Source: CAD feature listing. Evaluate the final solid. Frame: model axes, mm. Face numbers are marked on the shaded views. A direction names the side the tool comes from. Coordinates: 2 decimals unless noted, no trailing zeros. Loops run counter-clockwise (first coordinate to the right, second up) from the corner with the lowest first, then second, coordinate; pieces in that order, holes last. Notation, with made-up numbers: (71, 41.25) -> (85, 41.25) arc R10 cw to (85, 50.25) -> close; hole circle Ø8 at (22, 17). An arc over 180 degrees is marked (long way). One line per question, with ' | ' between items. Start each with the question number.
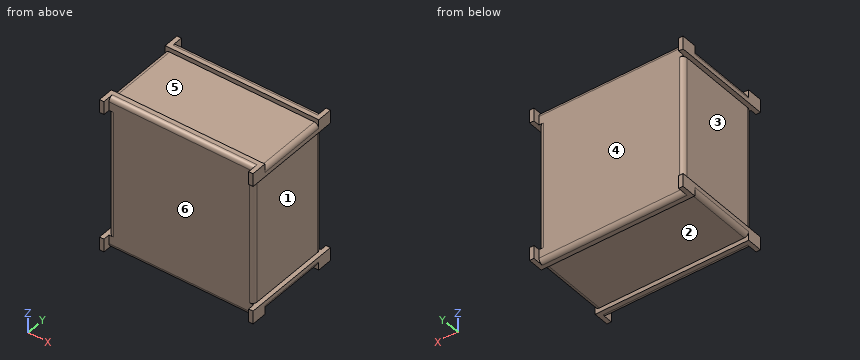
```python
from build123d import *

# Parameters (mm, degrees)
BOSS_EXTRUDE1_DEPTH = 23
CUT_EXTRUDE1_DEPTH  = 1.5
CUT_EXTRUDE2_DEPTH  = 1.5
FILLET2_R           = 1
FILLET3_R           = 1
FILLET4_R           = 1
FILLET5_R           = 1
CUT_EXTRUDE3_DEPTH  = 1
FILLET6_R           = 1
FILLET7_R           = 1
SKETCH6_W           = 35
SKETCH6_H           = 16.000000000000004
CUT_EXTRUDE4_DEPTH  = 1
FILLET8_R           = 1
FILLET9_R           = 1
CUT_EXTRUDE5_DEPTH  = 1
CUT_EXTRUDE6_DEPTH  = 1
FILLET10_R          = 1
FILLET11_R          = 1
FILLET12_R          = 1
FILLET13_R          = 1


with BuildPart() as part:
    # Sketch1 → Boss-Extrude1 (new body)
    with BuildSketch(Plane(origin=(0, 0, 0), x_dir=(1, 0, 0), z_dir=(0, 1, 0))):
        Polygon((-13.200362647325472, 10.07479601087942), (21.799637352674534, 10.07479601087942), (21.799637352674537, -24.925203989120583), (-13.200362647325466, -24.925203989120583), align=None)
    extrude(amount=BOSS_EXTRUDE1_DEPTH)

    # Sketch2 → Cut-Extrude1 (cut)
    with BuildSketch(Plane(origin=(0, 23, 0), x_dir=(1, 0, 0), z_dir=(0, 1, 0))):
        Polygon((20.79963735267453, -24.925203989120583), (-12.200362647325468, -24.925203989120586), (-12.20036264732547, 10.074796010879416), (20.79963735267453, 10.07479601087942), align=None)
    extrude(amount=-CUT_EXTRUDE1_DEPTH, mode=Mode.SUBTRACT)

    # Sketch3 → Cut-Extrude2 (cut)
    with BuildSketch(Plane.XZ):
        Polygon((20.799637352674537, -10.07479601087942), (-12.200362647325464, -10.074796010879423), (-12.200362647325463, 24.92520398912058), (20.799637352674537, 24.925203989120583), align=None)
    extrude(amount=-CUT_EXTRUDE2_DEPTH, mode=Mode.SUBTRACT)

    # Fillet2
    fillet2_edges = [part.edges().sort_by_distance(p)[0] for p in [
        (4.29963735267453, 21.5, -10.074796010879417),
    ]]
    fillet(fillet2_edges, radius=FILLET2_R)

    # Fillet3
    fillet3_edges = [part.edges().sort_by_distance(p)[0] for p in [
        (4.29963735267453, 21.5, 24.925203989120583),
    ]]
    fillet(fillet3_edges, radius=FILLET3_R)

    # Fillet4
    fillet4_edges = [part.edges().sort_by_distance(p)[0] for p in [
        (4.299637352674537, 1.5, 24.925203989120583),
    ]]
    fillet(fillet4_edges, radius=FILLET4_R)

    # Fillet5
    fillet5_edges = [part.edges().sort_by_distance(p)[0] for p in [
        (4.299637352674537, 1.5, -10.074796010879421),
    ]]
    fillet(fillet5_edges, radius=FILLET5_R)

    # Sketch5 → Cut-Extrude3 (cut)
    with BuildSketch(Plane(origin=(0, 0, -10.07479601087942), x_dir=(-1, 0, 0), z_dir=(0, 0, -1))):
        Polygon((13.200362647325472, 3.5089999999999977), (-21.799637352674534, 3.5089999999999937), (-21.799637352674534, 19.508999999999997), (13.200362647325472, 19.509), align=None)
    extrude(amount=-CUT_EXTRUDE3_DEPTH, mode=Mode.SUBTRACT)

    # Fillet6
    fillet6_edges = [part.edges().sort_by_distance(p)[0] for p in [
        (-13.200362647325472, 11.508999999999999, -9.07479601087942),
    ]]
    fillet(fillet6_edges, radius=FILLET6_R)

    # Fillet7
    fillet7_edges = [part.edges().sort_by_distance(p)[0] for p in [
        (21.799637352674534, 11.508999999999995, -9.07479601087942),
    ]]
    fillet(fillet7_edges, radius=FILLET7_R)

    # Sketch6 → Cut-Extrude4 (cut)
    with BuildSketch(Plane.XY.offset(24.925203989120583)):
        with Locations((4.299637352674536, 11.508999999999999)):
            Rectangle(SKETCH6_W, SKETCH6_H)
    extrude(amount=-CUT_EXTRUDE4_DEPTH, mode=Mode.SUBTRACT)

    # Fillet8
    fillet8_edges = [part.edges().sort_by_distance(p)[0] for p in [
        (-13.200362647325463, 11.509, 23.925203989120583),
    ]]
    fillet(fillet8_edges, radius=FILLET8_R)

    # Fillet9
    fillet9_edges = [part.edges().sort_by_distance(p)[0] for p in [
        (21.799637352674537, 11.508999999999999, 23.925203989120583),
    ]]
    fillet(fillet9_edges, radius=FILLET9_R)

    # Sketch7 → Cut-Extrude5 (cut)
    with BuildSketch(Plane(origin=(21.799637352674537, 0, -4.32e-15), x_dir=(-2e-16, 0, -1), z_dir=(1, 0, -2e-16))):
        Polygon((7.074796010879417, -1.2e-16), (-21.925203989120586, -3.95e-15), (-21.925203989120586, 22.999999999999996), (7.074796010879417, 22.999999999999996), align=None)
    extrude(amount=-CUT_EXTRUDE5_DEPTH, mode=Mode.SUBTRACT)

    # Sketch8 → Cut-Extrude6 (cut)
    with BuildSketch(Plane(origin=(-13.200362647325473, 0, -13.200362647325468), x_dir=(-1.5e-16, 0, -1), z_dir=(1, 0, -1.5e-16))):
        Polygon((-6.125566636446044, 8e-17), (-35.125566636446045, -3.47e-15), (-35.125566636446045, 22.999999999999996), (-6.1255666364460435, 23), align=None)
    extrude(amount=CUT_EXTRUDE6_DEPTH, mode=Mode.SUBTRACT)

    # Fillet10
    fillet10_edges = [part.edges().sort_by_distance(p)[0] for p in [
        (-12.20036264732547, 21.5, 7.425203989120572),
    ]]
    fillet(fillet10_edges, radius=FILLET10_R)

    # Fillet11
    fillet11_edges = [part.edges().sort_by_distance(p)[0] for p in [
        (-12.200362647325463, 1.5, 7.425203989120577),
    ]]
    fillet(fillet11_edges, radius=FILLET11_R)

    # Fillet12
    # the kernel refuses this fillet: 1 mm, written as the material it takes off along each edge
    with BuildSketch(Plane(origin=(20.79963735267453, 21.5, -7.074796010879421), x_dir=(-1, 0, 0), z_dir=(0, 0, 1))) as fillet12_piece_1:
        with BuildLine():
            CenterArc((FILLET12_R, FILLET12_R), FILLET12_R, 180, 90)
            Line((0, FILLET12_R), (0, 0))
            Line((0, 0), (FILLET12_R, 0))
        make_face()
    extrude(amount=29.000000000000004, mode=Mode.SUBTRACT)

    # Fillet13
    # the kernel refuses this fillet: 1 mm, written as the material it takes off along each edge
    with BuildSketch(Plane(origin=(20.799637352674537, 1.5, 21.925203989120583), x_dir=(-1, 0, 0), z_dir=(0, 0, -1))) as fillet13_piece_1:
        with BuildLine():
            CenterArc((FILLET13_R, FILLET13_R), FILLET13_R, 180, 90)
            Line((0, FILLET13_R), (0, 0))
            Line((0, 0), (FILLET13_R, 0))
        make_face()
    extrude(amount=29, mode=Mode.SUBTRACT)


solid = part.part
```
(1) Contact query for flat-ended pins moving along their axis: pin 1 Ø8 at (x, y) = (0.5, 8.5) entering from -Z; pin 2 Ø1.6 at (x, z) = (-1.5, -9.5) entering from -Y; pin 3 Ø5.5 at (y, z) = (10.5, 14.5) entering from -X. Output: stop coordinate, or through.
(2) Draft query along Y for the marked faces 3, 4, 5 and 6. Return one class per face: pulls with the +Y half, pulls with the -Y half, needs draft (parallel to the pull), parting line crosses it, or undercut.
(3) Cut plane B-B, the plane y = 3. Return the cut outline in (x, z).
(4) Access query for the marked faces 1 and 2. Directions: +Z, -Z, +X, -X, +Y, -Y. A direction counts if a zero-diameter tool reaches every point of the face in a straight line with its end or side. Return the directions, or none.
(5) Ray query, L1, parallel to X at y = 18.5, z = -1; L2, parallel to Z at x = 13, y = 7.5; L3, parallel to Y at x = 1, z = -5. Return the intervals inside material, ascending.
(6) Cut plane D-D, the plane y = 18. Return the cut outline in (x, z).
(7) Cut plane A-A, the plane x = 13. Return the cut outline in (y, z), and give its area (3 significant figures).
(8) Cut plane C-C, the plane z = 19.5. Return the cut outline in (x, y), and give its area (3 significant figures).
Here are the results:
1) pin 1: stops at z = -9.07 | pin 2: stops at y = 1.5 | pin 3: stops at x = -12.2
2) face 3: needs draft | face 4: pulls with the +Y half | face 5: undercut | face 6: pulls with the -Y half
3) outline: (-13.2, -10.07) -> (21.8, -10.07) -> (21.8, -7.07) -> (20.8, -7.07) -> (20.8, 21.93) -> (21.8, 21.93) -> (21.8, 24.93) -> (-13.2, 24.93) -> (-13.2, 21.93) -> (-12.2, 21.93) -> (-12.2, -7.07) -> (-13.2, -7.07) -> close
4) face 1: +X, +Y, -Y | face 2: -Z, +X, -X
5) L1: x = -12.2 to 20.8 | L2: z = -9.07 to 23.93 | L3: y = 1.5 to 21.5
6) outline: (-13.2, -8.07) arc R1 ccw to (-12.2, -9.07) -> (20.8, -9.07) arc R1 ccw to (21.8, -8.07) -> (21.8, -7.07) -> (20.8, -7.07) -> (20.8, 21.93) -> (21.8, 21.93) -> (21.8, 22.93) arc R1 ccw to (20.8, 23.93) -> (-12.2, 23.93) arc R1 ccw to (-13.2, 22.93) -> (-13.2, 21.93) -> (-12.2, 21.93) -> (-12.2, -7.07) -> (-13.2, -7.07) -> close
7) outline: (1.5, -9.07) arc R1 ccw to (2.5, -10.07) -> (3.51, -10.07) -> (3.51, -9.07) -> (19.51, -9.07) -> (19.51, -10.07) -> (20.5, -10.07) arc R1 ccw to (21.5, -9.07) -> (21.5, 23.93) arc R1 ccw to (20.5, 24.93) -> (19.51, 24.93) -> (19.51, 23.93) -> (3.51, 23.93) -> (3.51, 24.93) -> (2.5, 24.93) arc R1 ccw to (1.5, 23.93) -> close | area: 667 mm2
8) outline: (-12.2, 2.5) arc R1 ccw to (-11.2, 1.5) -> (19.8, 1.5) arc R1 ccw to (20.8, 2.5) -> (20.8, 20.5) arc R1 ccw to (19.8, 21.5) -> (-11.2, 21.5) arc R1 ccw to (-12.2, 20.5) -> close | area: 659 mm2
